```python
from build123d import *

# Parameters (mm, degrees)
F1_R     = 11.5
F1_R_2   = 10.5
F0_W     = 25
F0_H     = 25
F4_DEPTH = 5
F5_R     = 10.5
F6_DEPTH = 5.001


with BuildPart() as f3:
    # F3: sweep along a path in F2
    with BuildLine(Plane.YZ) as f3_path:
        Line((0, 8.3436881795), (-19.8769871225, 10.5584980885))
    # F1 (on face) → F3 (sweep)
    with BuildSketch(Plane.XZ):
        with Locations((-7.256067358, 8.3436881795)):
            Circle(F1_R)
        with Locations((-7.256067358, 8.3436881795)):
            Circle(F1_R_2, mode=Mode.SUBTRACT)
    sweep(path=f3_path.line)

    # F0 (on Front) → F4 (join)
    with BuildSketch(Plane.XZ):
        with Locations((-7.256067358, 8.3436881795)):
            Rectangle(F0_W, F0_H)
    extrude(amount=-F4_DEPTH)

    # F5 (on face) → F6 (cut, through all)
    with BuildSketch(Plane.XZ):
        with Locations((-7.256067358, 8.3436881795)):
            Circle(F5_R)
    extrude(amount=-F6_DEPTH, mode=Mode.SUBTRACT)


solid = f3.part
```
Design review of the part built by this model. Coordinates are the model's own, in mm. A direction names the side the tool comes from. Coordinates: 2 decimals unless noted, no trailing zeros. Answer as a JSON object with one key per item and string values. Group by question number.
1) Mouldability with a two-part tool opening along Z and no side actions: class faces 1 (the cylindrical face through (-1.611, 2.465, 17.197)), 2 (the flat face through (-7, 2, -4.156)), 3 (the flat face through (-12, -19.877, 1)) as pulls with the +Z half, pulls with the -Z half, needs draft (parallel to the pull), parting line crosses it, or undercut.
2) Wall thickness on L1, parallel to X at y = -1.75, z = 8.5; L2, parallel to Z at x = -13.5, y = -10.75; L3, parallel to Y at x = -14, z = 20: over which ranges is each line inside the solid? List them lowest first.
3) Tool access review of faces 4 (the flat face through (-7, 2, 20.844)), 5 (the flat face through (-17.5, 0, 14)), 6 (the flat face through (-19.756, 2, 8)): name each direction out of +Z, -Z, +X, -X, +Y, -Y from which nothing blocks a thin tool from reaching the whole face with its end or side.
4) For pin 1 (3 mm diameter, centred on x = -16.5, y = -11.5, fed in from -Z); pin 2 (3 mm diameter, centred on y = -6.5, z = 7.5, fed in from -X); pin 3 (1.5 mm diameter, centred on x = -6, y = 3, fed in from +Z); pin 4 (5 mm diameter, centred on x = 0.5, z = 1.5, fed in from -Y), all flat-tipped, find the tip position at first contact; note any pin that passes through.
Computed values:
{
 "1": {"face 1": "undercut", "face 2": "pulls with the -Z half", "face 3": "needs draft"},
 "2": {"L1": "x = -18.76 to -17.76, 3.24 to 4.24", "L2": "z = -0.12 to 1.1, 17.98 to 19.2", "L3": "y = 0 to 5"},
 "3": {"face 4": "+Z, +X, -X, +Y", "face 5": "none", "face 6": "+Z, -Z, -X, +Y, -Y"},
 "4": {"pin 1": "stops at z = 1.11", "pin 2": "stops at x = -18.76", "pin 3": "stops at z = 20.84", "pin 4": "stops at y = -19.88"}
}
